```python
from build123d import *

# Parameters (mm, degrees)
SKETCH_W     = 14.8
SKETCH_H     = 14.8
PAD_DEPTH    = 8
SKETCH001_R  = 2.9
PAD001_DEPTH = 3
FILLET_R     = 2
FILLET001_R  = 1


with BuildPart() as part:
    # Sketch → Pad (new body)
    with BuildSketch(Plane.XY):
        Rectangle(SKETCH_W, SKETCH_H)
    extrude(amount=PAD_DEPTH)

    # Sketch001 → Pad001 (new body)
    with BuildSketch(Plane(origin=(0, 0, 0), x_dir=(1, 0, 0), z_dir=(0, 0, -1))):
        with Locations((-7.4, 0)):
            Circle(SKETCH001_R)
        with Locations((7.4, 0)):
            Circle(SKETCH001_R)
    extrude(amount=-PAD001_DEPTH)

    # Fillet
    fillet_edges = [part.edges().sort_by_distance(p)[0] for p in [
        (7.4, 7.4, 4),
        (7.4, -7.4, 4),
        (-7.4, 7.4, 4),
        (-7.4, -7.4, 4),
    ]]
    fillet(fillet_edges, radius=FILLET_R)

    # Fillet001
    fillet001_edges = [part.edges().sort_by_distance(p)[0] for p in [
        (0, 7.4, 8),
        (6.814214, 6.814214, 8),
        (7.4, 0, 8),
        (6.814214, -6.814214, 8),
        (0, -7.4, 8),
        (-6.814214, -6.814214, 8),
        (-7.4, 0, 8),
        (-6.814214, 6.814214, 8),
    ]]
    fillet(fillet001_edges, radius=FILLET001_R)


solid = part.part
```
Input: part model. Units: mm. Frame: model coordinates. A direction names the side the tool comes from. Coordinates: 2 decimals unless noted, no trailing zeros. Write each loop counter-clockwise with the first axis right and the second up, starting at its lowest first coordinate (ties: lowest second). Pieces come first, ordered by that corner, then holes. Notation, with made-up numbers: M 68,35 L 103,35 A22 cw 103,58 Z; hole C 7.5,34 d8. An arc over 180 degrees is marked long. Use one line per item in the form item = value.
Q1. Set-up query: faces 1 (the face through (-9, 0, 3)), 2 (the face through (7.4, 0, 4)), 3 (the face through (-7.4, 0, 4)). Return all of +Z, -Z, +X, -X, +Y, -Y with unobstructed straight access to the full face (end or side cutting, diameter ignored); none if empty.
Answer below:
face_1 = +Z, -X, +Y, -Y
face_2 = +Z, +X
face_3 = +Z, -X
Q2. Section B-B (z = 3.75). Return loops of the section in (x, y).
Answer below:
outline = M -7.4,-5.4 A2 ccw -5.4,-7.4 L 5.4,-7.4 A2 ccw 7.4,-5.4 L 7.4,5.4 A2 ccw 5.4,7.4 L -5.4,7.4 A2 ccw -7.4,5.4 Z
Q3. Section C-C (y = 3.5). Return loops of the section in (x, z).
Answer below:
outline = M -7.4,0 L 7.4,0 L 7.4,7 A1 ccw 6.4,8 L -6.4,8 A1 ccw -7.4,7 Z
Q4. Material intervals for probe 1 along Z at (x, y) = (9, 1); probe 2 along X at (y, z) = (-3, 6); probe 3 along X at (y, z) = (-6.25, 6), sorted ascending. Write a range as from..to.
Answer below:
probe_1 = 0..3
probe_2 = -7.4..7.4
probe_3 = -7.21..7.21
Q5. Section D-D (x = -9). Return loops of the section in (y, z).
Answer below:
outline = M -2.42,0 L 2.42,0 L 2.42,3 L -2.42,3 Z
Q6. First-contact query: pin 1 (1.5 mm diameter, centred on x = -9, y = -1, fed in from +Z); pin 2 (2 mm diameter, centred on y = 0.5, z = 2, fed in from +X). Flat tips, straight axial feed; report the tip coordinate or a pass-through.
Answer below:
pin_1 = 3
pin_2 = 10.3
Q7. Section A-A (y = 0). Return loops of the section in (x, z).
Answer below:
outline = M -10.3,0 L 10.3,0 L 10.3,3 L 7.4,3 L 7.4,7 A1 ccw 6.4,8 L -6.4,8 A1 ccw -7.4,7 L -7.4,3 L -10.3,3 Z
